```python
from build123d import *

# Parameters (mm, degrees)
F0_W     = 10
F0_H     = 3
F0_R     = 1.75
F1_DEPTH = 3


with BuildPart() as f1:
    # F0 (on Right) → F1 (new body)
    with BuildSketch(Plane.YZ):
        Polygon((10, -42), (10, 42), (5, 42), (-5, 42), (-10, 42), (-10, -42), (-5, -42), (5, -42), align=None)
        with Locations((0, -37.5)):
            Rectangle(F0_W, F0_H, mode=Mode.SUBTRACT)
        with Locations((0, -22)):
            Circle(F0_R, mode=Mode.SUBTRACT)
        with Locations((0, 22)):
            Circle(F0_R, mode=Mode.SUBTRACT)
        with Locations((0, 37.5)):
            Rectangle(F0_W, F0_H, mode=Mode.SUBTRACT)
        with Locations((0, 43.5)):
            Rectangle(F0_W, F0_H)
        with Locations((0, -43.5)):
            Rectangle(F0_W, F0_H)
    extrude(amount=F1_DEPTH)


solid = f1.part
```
Design review of the part built by this model. Coordinates are the model's own, in mm. A direction names the side the tool comes from. Coordinates: 2 decimals unless noted, no trailing zeros. Order: outer loops, then holes, each group sorted by start corner. A loop starts at its lowest first (then second) coordinate and runs counter-clockwise, first axis right, second up. Notation, with made-up numbers: (7, 18.25) - (25, 18.25) arc R22 ccw to (25, 52.25) - close; hole circle Ø4 at (65.25, -39). An arc over 180 degrees is marked (long way). Answer in a Markdown table with one row per item.
(1) For faces 1 (the flat face through (1, 5, 37)), 2 (the flat face through (1, -7, 42)), 3 (the flat face through (1, -10, 1)), 4 (the flat face through (1, 8, 42)), 5 (the flat face through (1, -8, -42)), list the 3-axis set-ups (+Z, -Z, +X, -X, +Y, -Y) from which the entire face can be reached by the end or side of a thin tool; tool diameter is ignored.
Checked values:
| item | result |
|---|---|
| face 1 | +X, -X |
| face 2 | +Z, +X, -X, -Y |
| face 3 | +Z, -Z, +X, -X, -Y |
| face 4 | +Z, +X, -X, +Y |
| face 5 | -Z, +X, -X, -Y |
(2) Consider section D-D on y = 7. State the section outline as (x, z) points.
Checked values:
| item | result |
|---|---|
| outline | (0, -42) - (3, -42) - (3, 42) - (0, 42) - close |
(3) Consider section C-C on x = 0.75. State the section outline as (y, z) points, plus the area to 3 significant figures.
Checked values:
| item | result |
|---|---|
| outline | (-10, -42) - (-5, -42) - (-5, -45) - (5, -45) - (5, -42) - (10, -42) - (10, 42) - (5, 42) - (5, 45) - (-5, 45) - (-5, 42) - (-10, 42) - close; hole (-5, -39) - (5, -39) - (5, -36) - (-5, -36) - close; hole (-5, 36) - (5, 36) - (5, 39) - (-5, 39) - close; hole circle Ø3.5 at (0, -22); hole circle Ø3.5 at (0, 22) |
| area | 1,660 mm^2 |
(4) The part is to be moulded in two halves that separate along Y. For faces 6 (the flat face through (1, -5, 43)), 7 (the flat face through (1, 10, -1)), 8 (the cylindrical face through (1.479, -0.228, 23.735)), say which applies: released by +Y, released by -Y, zero draft, split by the parting line, or undercut.
Checked values:
| item | result |
|---|---|
| face 6 | released by -Y |
| face 7 | released by +Y |
| face 8 | undercut |
(5) Wall thickness on line 1 along Z through (x, y) = (1.05, -2.5); line 2 along Z through (x, y) = (1.45, 0); line 3 along Y through (x, z) = (2.05, 36.5): over which ranges is each line inside the solid? List them lowest first. Write a range as from..to.
Checked values:
| item | result |
|---|---|
| line 1 | -45..-39, -36..36, 39..45 |
| line 2 | -45..-39, -36..-23.75, -20.25..20.25, 23.75..36, 39..45 |
| line 3 | -10..-5, 5..10 |
(6) Clearance check with flat-ended pins moving along their axes: pin 1 (3 mm diameter, centred on y = 0, z = -22, fed in from -X); pin 2 (1.5 mm diameter, centred on x = 1, y = 8, fed in from -Z); pin 3 (0.9 mm diameter, centred on x = 1.5, z = -44, fed in from +Y); pin 4 (1.5 mm diameter, centred on x = 2, z = -44, fed in from -Y). State where each tip first meets the part, or that it passes through.
Checked values:
| item | result |
|---|---|
| pin 1 | through |
| pin 2 | z = -42 |
| pin 3 | y = 5 |
| pin 4 | y = -5 |
(7) Consider section A-A on y = 0. State the section outline as (x, z) points.
Checked values:
| item | result |
|---|---|
| outline | (0, -45) - (3, -45) - (3, -39) - (0, -39) - close; (0, -36) - (3, -36) - (3, -23.75) - (0, -23.75) - close; (0, -20.25) - (3, -20.25) - (3, 20.25) - (0, 20.25) - close; (0, 23.75) - (3, 23.75) - (3, 36) - (0, 36) - close; (0, 39) - (3, 39) - (3, 45) - (0, 45) - close |
(8) Consider section B-B on z = 22. State the section outline as (x, y) points, plus the area to 3 significant figures.
Checked values:
| item | result |
|---|---|
| outline | (0, -10) - (3, -10) - (3, -1.75) - (0, -1.75) - close; (0, 1.75) - (3, 1.75) - (3, 10) - (0, 10) - close |
| area | 49.5 mm^2 |
